For this review, take the finished solid that the model builds, in its own axes (mm). Face numbers are marked on the shaded views. Coordinates: 2 decimals unless noted, no trailing zeros. Write each loop counter-clockwise with the first axis right and the second up, starting at its lowest first coordinate (ties: lowest second). Pieces come first, ordered by that corner, then holes. Notation, with made-up numbers: (6.5, 84.5) -> (15.5, 84.5) arc R25 ccw to (15.5, 97.5) -> close; hole circle Ø6 at (64, 87). An arc over 180 degrees is marked (long way). One line per item, written item: value. Start each with the question number.
1) Add section A-A (y = -1.5). State the section outline as (x, z) points.
2) Mouldability with a two-part tool opening along Y and no side actions: class the marked faces 1, 2, 3 and 4 as released by +Y, released by -Y, zero draft, split by the parting line, or undercut.
3) Add section C-C (z = 0.4). State the section outline as (x, y) points.
4) Add section B-B (x = 0.6). State the section outline as (y, z) points, and give its area (3 significant figures).
5) For probe 1 along Y at (x, z) = (-2.45, 1.1); probe 2 along X at (y, z) = (3, 1.2); probe 3 along X at (y, z) = (-0.5, 1.35), list the stretches that pass through material, from the lowest coordinate up. Write a range as from..to.
6) For pin 1 Ø0.8 at (x, z) = (-0.5, 1) entering from -Y, flat-tipped, find the tip position at first contact; note if it passes through.
7) Add section D-D (y = 2.5). State the section outline as (x, z) points.
Autodesk Inventor part; units mm, degrees
ref_plane "YZ Plane" through (0, 0, 0) normal (1, 0, 0) x (0, 1, 0)
ref_plane "XZ Plane" through (0, 0, 0) normal (0, 1, 0) x (-1, 0, 0)
ref_plane "XY Plane" through (0, 0, 0) normal (0, 0, 1) x (1, 0, 0)
sketch "Sketch1" plane through (0, 0, 0) normal (1, 0, 0) x (0, 1, 0)
  point P0 (0, 0)
sketch "Sketch2" plane through (0, 0, 0) normal (0, 0, 1) x (1, 0, 0)
  line L0 (4.0785, 4.9113) -> (2.4908, 4.9113) construction
  line L1 (4.0785, 3.7037) -> (4.0785, 4.9113) construction
  line L2 (2.4323, 3.7037) -> (4.0785, 3.7037) construction
  arc A0 (2.4323, 3.7037) -> (2.2344, -2.9627) centre (6.1869, 0.2561) ccw
  arc A1 (1.8925, -3.3998) -> (2.2344, -2.9627) centre (2.0138, -3.1424) ccw
  arc A2 (-0.5696, -0.5268) -> (1.8925, -3.3998) centre (3.8604, 0.7782) ccw
  line L3 (-1.0058, 0.9542) -> (-0.5696, -0.5268)
  arc A3 (-1.0058, 0.9542) -> (-0.2339, -2.7516) centre (2.2087, -0.3095) ccw
  arc A4 (-0.2339, -2.7516) -> (1.9052, -3.655) centre (1.9474, -0.5708) ccw
  line L4 (2.5244, -3.655) -> (1.9052, -3.655) construction
  line L5 (2.5244, -4.0286) -> (2.5244, -3.655) construction
  line L6 (1.9895, -4.0228) -> (2.5244, -4.0286) construction
  line L7 (1.9895, -3.8389) -> (1.9895, -4.0228) construction
  line L8 (1.9474, -3.8389) -> (1.9895, -3.8389) construction
  arc A5 (0.288, -3.3863) -> (1.9474, -3.8389) centre (1.9474, -0.5708) ccw construction
  line L9 (-3.5298, -3.3863) -> (0.288, -3.3863) construction
  line L10 (-3.5298, 3.7037) -> (-3.5298, -3.3863) construction
  line L11 (1.3533, 3.7037) -> (-3.5298, 3.7037) construction
  line L12 (2.4908, 4.9113) -> (1.3533, 3.7037) construction
  line L13 (0.288, -3.3863) -> (0.6877, -3.3863)
  line L14 (2.4323, 3.7037) -> (-3.5298, 3.7037)
  line L15 (-3.5298, -3.3863) -> (-3.5298, 3.7037)
  line L16 (0.288, -3.3863) -> (-3.5298, -3.3863)
  point P0 (0, 0)
extrude "Plate1" add sketch "Sketch2" along normal blind 1.5
equation "\"d0\" = Thickness"
equation "\"BendRadius\" = Thickness"
equation "\"BendReliefWidth\" = Thickness"
equation "\"BendReliefDepth\" = 0.5 * Thickness"
equation "\"CornerReliefSize\" = 4 * Thickness"
equation "\"MinimumRemnant\" = 2 * Thickness"
equation "\"TransitionRadius\" = BendRadius"
equation "\"JacobiRadiusSize\" = BendRadius"
equation "\"GapSize\" = Thickness"
properties part number "TRIGGER_2"
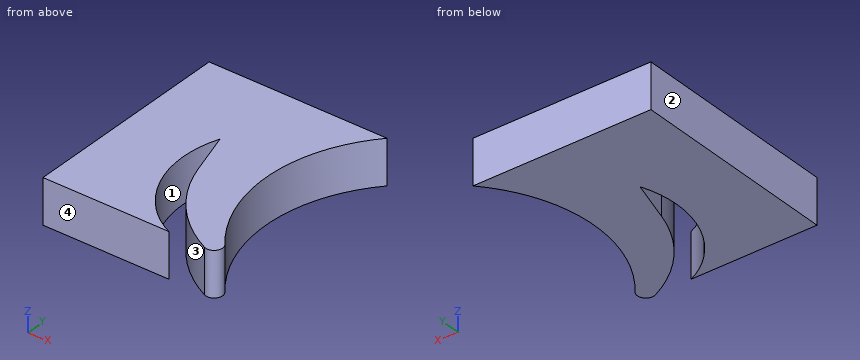
Numbers:
1. outline: (-3.53, 0) -> (-1.03, 0) -> (-1.03, 1.5) -> (-3.53, 1.5) -> close; (-0.16, 0) -> (1.4, 0) -> (1.4, 1.5) -> (-0.16, 1.5) -> close
2. face 1: undercut
2. face 2: zero draft
2. face 3: undercut
2. face 4: released by -Y
3. outline: (-3.53, -3.39) -> (0.69, -3.39) arc R3.08 cw to (-0.23, -2.75) arc R3.45 cw to (-1.01, 0.95) -> (-0.57, -0.53) arc R4.62 ccw to (1.89, -3.4) arc R0.28 ccw to (2.23, -2.96) arc R5.1 cw to (2.43, 3.7) -> (-3.53, 3.7) -> close
4. outline: (-3.39, 0) -> (-3.35, 0) -> (-3.35, 1.5) -> (-3.39, 1.5) -> close; (-2.49, 0) -> (3.7, 0) -> (3.7, 1.5) -> (-2.49, 1.5) -> close
4. area: 9.36 mm²
5. probe 1: -3.39..3.7
5. probe 2: -3.53..1.89
5. probe 3: -3.53..-1.24, -0.58..1.15
6. pin 1: y = -3.39
7. outline: (-3.53, 0) -> (1.61, 0) -> (1.61, 1.5) -> (-3.53, 1.5) -> close
